Print and shaded views of the part. All mm, measured from the part's lowest x, y and z. A direction names the side the tool comes from. Round coordinates to 2 decimals unless told otherwise and drop trailing zeros. Write each loop counter-clockwise with the first axis right and the second up, starting at its lowest first coordinate (ties: lowest second). Pieces come first, ordered by that corner, then holes. Notation, with made-up numbers: M -20,26.5 L 31,26.5 A12 cw 31,46.5 Z; hole C 34.25,61.25 d4. An arc over 180 degrees is marked long. Write item = value, one per line.
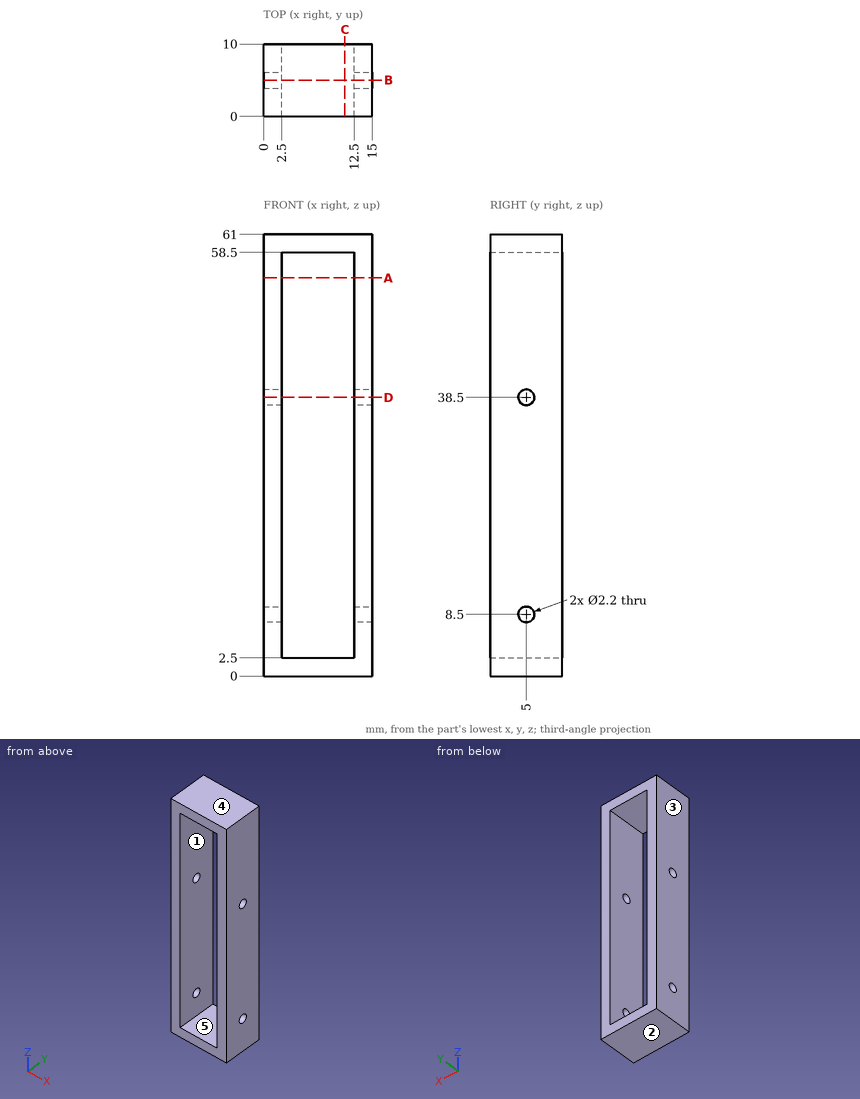
1. Probe probe 1 along Z at (x, y) = (14.25, 5); probe 2 along X at (y, z) = (4.5, 51.5); probe 3 along Z at (x, y) = (5.5, 7.75). List the from-to ranges inside material, lowest first.
Responses:
probe_1 = 0 to 7.4, 9.6 to 37.4, 39.6 to 61
probe_2 = 0 to 2.5, 12.5 to 15
probe_3 = 0 to 2.5, 58.5 to 61
2. Flat gauge pin, fed straight in: pin 1 (2.5 mm diameter, centred on y = 5, z = 8.5, fed in from -X). Where does the tip first touch, or does it go through?
Responses:
pin_1 = 0
3. Tool access for the marked faces 4 and 5: list every direction of +Z, -Z, +X, -X, +Y, -Y with a clear straight run to the whole face (end or side of a thin tool).
Responses:
face_4 = +Z, +X, -X, +Y, -Y
face_5 = +Y, -Y
4. Band-saw the part on D-D (z = 38.5). List the corners of the cut face in (x, y).
Responses:
outline = M 0,0 L 2.5,0 L 2.5,3.9 L 0,3.9 Z; M 0,6.1 L 2.5,6.1 L 2.5,10 L 0,10 Z; M 12.5,0 L 15,0 L 15,3.9 L 12.5,3.9 Z; M 12.5,6.1 L 15,6.1 L 15,10 L 12.5,10 Z
5. Band-saw the part on A-A (z = 55). List the corners of the cut face in (x, y), plus the area to 3 significant figures.
Responses:
outline = M 0,0 L 2.5,0 L 2.5,10 L 0,10 Z; M 12.5,0 L 15,0 L 15,10 L 12.5,10 Z
area = 50.0 mm²
6. Band-saw the part on C-C (x = 11.25). List the corners of the cut face in (y, z).
Responses:
outline = M 0,0 L 10,0 L 10,2.5 L 0,2.5 Z; M 0,58.5 L 10,58.5 L 10,61 L 0,61 Z
7. Mould opens along X. For the marked faces 1, 2 and 3 say: pulls with the +X half, pulls with the -X half, needs draft (parallel to the pull), parting line crosses it, or undercut.
Responses:
face_1 = undercut
face_2 = needs draft
face_3 = pulls with the -X half
8. Band-saw the part on B-B (y = 5). List the corners of the cut face in (x, z).
Responses:
outline = M 0,0 L 15,0 L 15,7.4 L 12.5,7.4 L 12.5,2.5 L 2.5,2.5 L 2.5,7.4 L 0,7.4 Z; M 0,9.6 L 2.5,9.6 L 2.5,37.4 L 0,37.4 Z; M 0,39.6 L 2.5,39.6 L 2.5,58.5 L 12.5,58.5 L 12.5,39.6 L 15,39.6 L 15,61 L 0,61 Z; M 12.5,9.6 L 15,9.6 L 15,37.4 L 12.5,37.4 Z
